Source: three-view drawing plus pictorial views. Frame: mm from the lowest corner of the part. Give positions to 0.01 mm unless a question says otherwise; leave off trailing zeros. Write each loop counter-clockwise with the first axis right and the second up, starting at its lowest first coordinate (ties: lowest second). Pieces come first, ordered by that corner, then holes.
Q1. Cut plane B-B on z = 25.5. Return the cut outline in (x, y) (1 decimal).
Q2. Line query: L1, parallel to X at y = 5.75, z = 46.5 (1 decimal); L2, parallel to X at y = 7, z = 39.5 (1 decimal); L3, parallel to Y at x = 2, z = 12. Output: solid intervals per line, ascending.
Q3. Pin query (flat end, axial travel): pin 1 (5 mm diameter, centred on x = 5.5, y = 3, fed in from -Z); pin 2 (1 mm diameter, centred on x = 0.5, z = 61, fed in from +Y); pin 3 (3 mm diameter, centred on y = 4, z = 36, fed in from +X); pin 4 (1 mm diameter, centred on y = 7.5, z = 37.5, fed in from -X) (3 decimals). Return the tip coordinate at first contact, or that it passes through.
Q4. Cut plane C-C on x = 9.5. Return the cut outline in (y, z), plus the area to 3 significant figures.
Q5. Cut plane D-D on z = 10. Return the cut outline in (x, y), plus the area to 3 significant figures.
Q6. Cut plane A-A on y = 6. Return the cut outline in (x, z) (1 decimal), plus the area to 3 significant figures.
Q7. Draft query along Z for the marked faces 1, 2 and 3. Return one class per face: pulls with the +Z half, pulls with the -Z half, needs draft (parallel to the pull), parting line crosses it, or undercut.
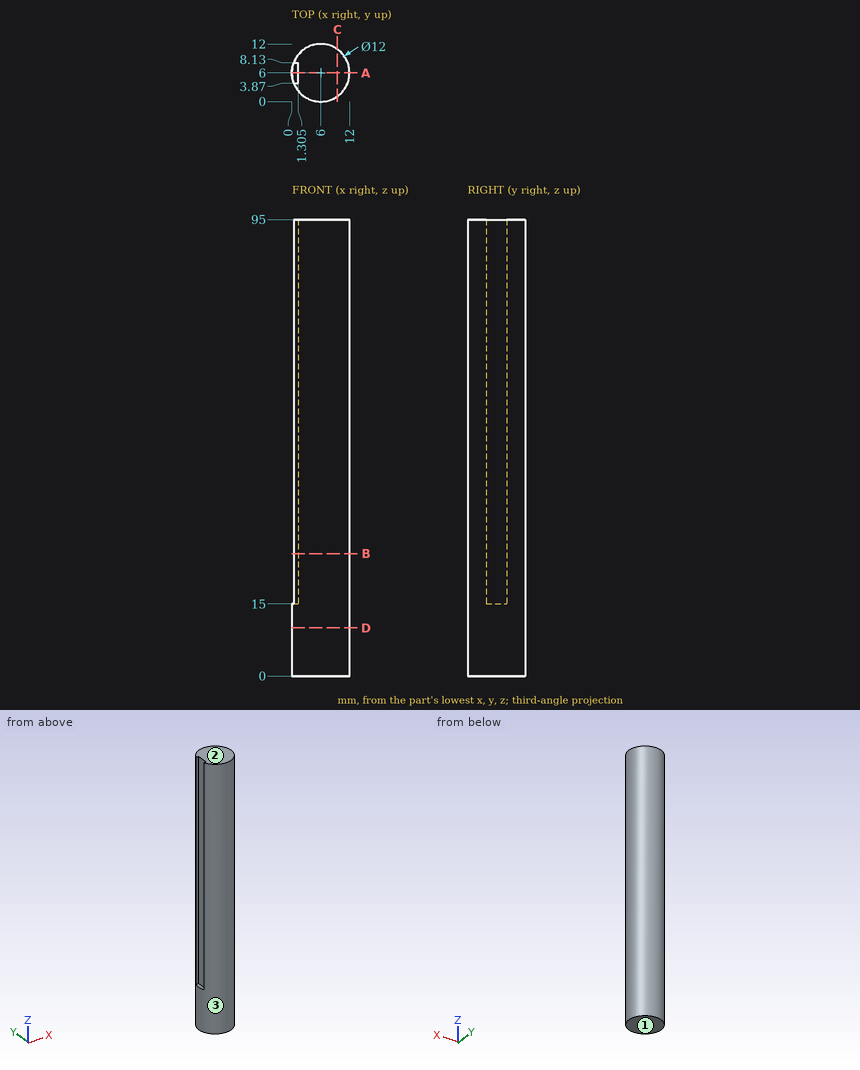
Data:
1. outline: (0.4, 3.9) arc R6 ccw (long way) to (0.4, 8.1) - (1.3, 8.1) - (1.3, 3.9) - close
2. L1: x = 1.3 to 12
2. L2: x = 1.3 to 11.9
2. L3: y = 1.53 to 10.47
3. pin 1: stops at z = 0
3. pin 2: stops at y = 9.32
3. pin 3: stops at x = 11.98
3. pin 4: stops at x = 1.305
4. outline: (1.13, 0) - (10.87, 0) - (10.87, 95) - (1.13, 95) - close
4. area: 926 mm2
5. outline: circle Ø12 at (6, 6)
5. area: 113 mm2
6. outline: (0, 0) - (12, 0) - (12, 95) - (1.3, 95) - (1.3, 15) - (0, 15) - close
6. area: 1,040 mm2
7. face 1: pulls with the -Z half
7. face 2: pulls with the +Z half
7. face 3: needs draft
